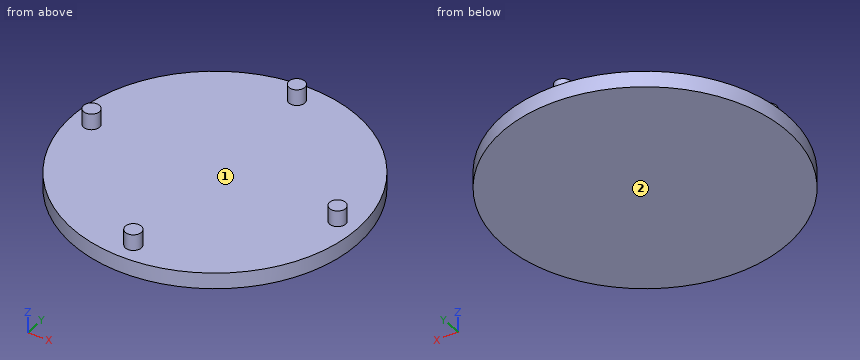
```python
from build123d import *

# Parameters (mm, degrees)
F0_R     = 15.875
F1_DEPTH = 1.778
F3_R     = 0.889
F4_DEPTH = 1.778


with BuildPart() as f1:
    # F0 (on Top) → F1 (new body)
    with BuildSketch(Plane.XY):
        Circle(F0_R)
    extrude(amount=-F1_DEPTH)

    # F3 (on face) → F4 (join)
    with BuildSketch(Plane.XY):
        with Locations((0, 13.652203)):
            Circle(F3_R)
        with Locations((-13.659894, -0.015021)):
            Circle(F3_R)
        with Locations((0.062219, -13.682245)):
            Circle(F3_R)
        with Locations((13.674476, -0.124876)):
            Circle(F3_R)
    extrude(amount=F4_DEPTH)


solid = f1.part
```
The listing builds one solid part. Answer for the finished solid, in the listing's coordinates (mm). Face numbers are marked on the shaded views. A direction names the side the tool comes from. Coordinates: 2 decimals unless noted, no trailing zeros. Loops run counter-clockwise (first coordinate to the right, second up) from the corner with the lowest first, then second, coordinate; pieces in that order, holes last. Notation, with made-up numbers: M -4.75,20 L 25.25,20 A22 ccw 25.25,57 Z; hole C 34,36.5 d5. An arc over 180 degrees is marked long. Answer as a JSON object with one key per item and string values. Group by question number.
Item 1: Consider L1, parallel to Z at x = -14, y = -6.5; L2, parallel to X at y = 0.5, z = 1.1; L3, parallel to Y at x = 0.5, z = -0.25. Determine where each line is inside the solid, lowest interval first.
Item 2: Each of these flat-tipped pins is pushed along its axis until it touches: P1, Ø12, axis at x = 12, y = -10, coming from the +Z side; P2, Ø2, axis at x = -7, z = -1.5, coming from the -Y side. Where does it stop, or does it pass through?
Item 3: Section A-A (x = 0) is taken. Write down the section's boundary in (y, z) (3 decimals), and give its area (3 significant figures).
Item 4: Section B-B (y = -0.5) is taken. Write down the section's boundary in (x, z), and give its area (3 significant figures).
Item 5: Which of the six approach directions +Z, -Z, +X, -X, +Y, -Y give full straight-line access (tool end or side, diameter ignored) to the marked faces 1 and 2?
Item 6: Section C-C (z = 1.15) is taken. Write down the section's boundary in (x, y).
Item 7: Section D-D (y = 10) is taken. Write down the section's boundary in (x, z).
Solved:
{
 "1": {"L1": "z = -1.78 to 0", "L2": "x = -14.38 to -12.94, 13.04 to 14.31", "L3": "y = -15.87 to 15.87"},
 "2": {"P1": "stops at z = 0", "P2": "stops at y = -14.7"},
 "3": {"outline": "M -15.875,-1.778 L 15.875,-1.778 L 15.875,0 L 14.541,0 L 14.541,1.778 L 12.763,1.778 L 12.763,0 L -12.795,0 L -12.795,1.778 L -14.569,1.778 L -14.569,0 L -15.875,0 Z", "area": "62.8 mm2"},
 "4": {"outline": "M -15.87,-1.78 L 15.87,-1.78 L 15.87,0 L 14.48,0 L 14.48,1.78 L 12.87,1.78 L 12.87,0 L -12.91,0 L -12.91,1.78 L -14.4,1.78 L -14.4,0 L -15.87,0 Z", "area": "61.9 mm2"},
 "5": {"face 1": "+Z", "face 2": "-Z, +X, -X, +Y, -Y"},
 "6": {"outline": "C -13.66,-0.02 d1.78; C 0,13.65 d1.78; C 0.06,-13.68 d1.78; C 13.67,-0.12 d1.78"},
 "7": {"outline": "M -12.33,-1.78 L 12.33,-1.78 L 12.33,0 L -12.33,0 Z"}
}
